```python
from build123d import *

# Parameters (mm, degrees)
F0_W     = 609.6
F0_H     = 762
F1_DEPTH = 304.8
F2_W     = 571.5
F2_H     = 361.95
F3_DEPTH = 285.75
F5_DEPTH = 762
F6_W     = 304.8
F6_H     = 19.05
F7_DEPTH = 1079.5


with BuildPart() as f1:
    # F0 (on Front) → F1 (new body)
    with BuildSketch(Plane.XZ):
        Rectangle(F0_W, F0_H)
    extrude(amount=F1_DEPTH)

    # F2 (on face) → F3 (cut, through all)
    with BuildSketch(Plane.XZ.offset(304.8)):
        with Locations((0, 200.025)):
            Rectangle(F2_W, F2_H)
        with Locations((0, -180.975)):
            Rectangle(F2_W, F2_H)
    extrude(amount=-F3_DEPTH, mode=Mode.SUBTRACT)

    # F4 (on face) → F5 (join, through all)
    with BuildSketch(Plane.XY.offset(381)):
        Polygon((285.75, 0), (304.8, 0), (304.8, 1524), (-304.8, 1524), (-304.8, 1504.95), (285.75, 1504.95), (285.75, 425.45), (-19.05, 425.45), (-19.05, 387.35), (285.75, 387.35), align=None)
    extrude(amount=-F5_DEPTH)

    # F6 (on face) → F7 (join, through all)
    with BuildSketch(Plane.XZ.offset(-1504.95)):
        with Locations((133.35, -269.875)):
            Rectangle(F6_W, F6_H)
        with Locations((133.35, 60.325)):
            Rectangle(F6_W, F6_H)
    extrude(amount=F7_DEPTH)


solid = f1.part
```
Part model, mm, in its own coordinate system. A direction names the side the tool comes from. Round coordinates to 2 decimals unless told otherwise and drop trailing zeros. Loops run counter-clockwise (first coordinate to the right, second up) from the corner with the lowest first, then second, coordinate; pieces in that order, holes last. Notation, with made-up numbers: (30, 12) -> (51, 12) arc R23 cw to (51, 36) -> close; hole circle Ø7 at (35.5, -38.5). An arc over 180 degrees is marked (long way). Use a Markdown table: item, result.
1) Drop flat-ended pins along their axis: pin 1 Ø8 at (x, y) = (239, 1239.5) entering from +Z; pin 2 Ø3 at (y, z) = (1255.5, 90) entering from -X; pin 3 Ø1 at (x, y) = (241, 1327) entering from -Z. Give the stop position or say it passes through.
The answers:
| item | result |
|---|---|
| pin 1 | stops at z = 69.85 |
| pin 2 | stops at x = 285.75 |
| pin 3 | stops at z = -279.4 |
2) Pull direction Y, two halves, no side cores. Call faces 6 (the flat face through (-4, -164, 19.05)), 7 (the flat face through (285.75, 196, 5)), 8 (the flat face through (-4, -19.05, 203)), 9 (the flat face through (-14, 0, 5)): pulls with the +Y half, pulls with the -Y half, needs draft (parallel to the pull), parting line crosses it, or undercut.
The answers:
| item | result |
|---|---|
| face 6 | needs draft |
| face 7 | undercut |
| face 8 | pulls with the -Y half |
| face 9 | undercut |
3) Cut at C-C, the plane y = 1191. List the corners of the cut face in (x, z), and give its area (3 significant figures).
The answers:
| item | result |
|---|---|
| outline | (-19.05, -279.4) -> (285.75, -279.4) -> (285.75, -381) -> (304.8, -381) -> (304.8, 381) -> (285.75, 381) -> (285.75, 69.85) -> (-19.05, 69.85) -> (-19.05, 50.8) -> (285.75, 50.8) -> (285.75, -260.35) -> (-19.05, -260.35) -> close |
| area | 26,100 mm2 |
4) Cut at A-A, the plane x = -98. List the corners of the cut face in (y, z), and give its area (3 significant figures).
The answers:
| item | result |
|---|---|
| outline | (-304.8, -381) -> (0, -381) -> (0, 381) -> (-19.05, 381) -> (-19.05, 19.05) -> (-304.8, 19.05) -> (-304.8, 0) -> (-19.05, 0) -> (-19.05, -361.95) -> (-304.8, -361.95) -> close; (1504.95, -381) -> (1524, -381) -> (1524, 381) -> (1504.95, 381) -> close |
| area | 39,900 mm2 |
5) Tool access for faces 1 (the flat face through (-285.75, -164, 197)), 2 (the flat face through (285.75, 973, -103)), 3 (the flat face through (-285.75, -164, -184)), 4 (the flat face through (131, 387.35, 5)), 5 (the flat face through (135, 425.45, 228)): list every direction of +Z, -Z, +X, -X, +Y, -Y with a clear straight run to the whole face (end or side of a thin tool).
The answers:
| item | result |
|---|---|
| face 1 | +Z, -Y |
| face 2 | -X |
| face 3 | -Y |
| face 4 | +Z, -Z, -X |
| face 5 | +Z, -X |
6) Cut at B-B, the plane x = 172. List the corners of the cut face in (y, z).
The answers:
| item | result |
|---|---|
| outline | (-304.8, -381) -> (0, -381) -> (0, 381) -> (-19.05, 381) -> (-19.05, 19.05) -> (-304.8, 19.05) -> (-304.8, 0) -> (-19.05, 0) -> (-19.05, -361.95) -> (-304.8, -361.95) -> close; (387.35, -381) -> (425.45, -381) -> (425.45, -279.4) -> (1504.95, -279.4) -> (1504.95, -381) -> (1524, -381) -> (1524, 381) -> (1504.95, 381) -> (1504.95, 69.85) -> (425.45, 69.85) -> (425.45, 381) -> (387.35, 381) -> close; hole (425.45, -260.35) -> (1504.95, -260.35) -> (1504.95, 50.8) -> (425.45, 50.8) -> close |
7) Probe line 1 (Y direction, x = 106, z = -90); line 2 (Y direction, x = -118.5, z = -116); line 3 (X direction, y = -211.5, z = -180). List the from-to ranges inside material, lowest first. Write a range as [from, to].
The answers:
| item | result |
|---|---|
| line 1 | y = [-19.05, 0], [387.35, 425.45], [1504.95, 1524] |
| line 2 | y = [-19.05, 0], [1504.95, 1524] |
| line 3 | x = [-304.8, -285.75], [285.75, 304.8] |
8) Cut at D-D, the plane z = 157. List the corners of the cut face in (x, y).
The answers:
| item | result |
|---|---|
| outline | (-304.8, -304.8) -> (-285.75, -304.8) -> (-285.75, -19.05) -> (285.75, -19.05) -> (285.75, -304.8) -> (304.8, -304.8) -> (304.8, 1524) -> (-304.8, 1524) -> (-304.8, 1504.95) -> (285.75, 1504.95) -> (285.75, 425.45) -> (-19.05, 425.45) -> (-19.05, 387.35) -> (285.75, 387.35) -> (285.75, 0) -> (-304.8, 0) -> close |
